Check sheet for the modelled part. Datum: model origin and axes. Units: mm. A direction names the side the tool comes from. Round coordinates to 2 decimals unless told otherwise and drop trailing zeros. Write each loop counter-clockwise with the first axis right and the second up, starting at its lowest first coordinate (ties: lowest second). Pieces come first, ordered by that corner, then holes. Notation, with made-up numbers: (9, -19) - (40, -19) arc R20 cw to (40, 17) - close; hole circle Ø1 at (42.25, 40.25). An arc over 180 degrees is marked (long way). Answer as a JSON object with one key per item and string values. Group by question number.
Item 1: Release check for a two-part mould opening along X. For faces 3 (the flat face through (4.28, -7.28, 15.86)), 4 (the flat face through (4.16, 7.35, 15.86)) record: pulls with the +X half, pulls with the -X half, needs draft (parallel to the pull), parting line crosses it, or undercut.
Item 2: Set-up check for faces 1 (the flat face through (-4.16, -7.35, 15.86)), 2 (the cylindrical face through (4.896, 2.03, 5.719)): record each of +Z, -Z, +X, -X, +Y, -Y from which the full face is reachable in a straight line by a thin tool's end or side.
Item 3: Gauge pin test, flat ends, axial feed: P1, Ø6.5, axis at x = 0, y = 0, coming from the +Z side; P2, Ø3, axis at x = -21, z = 17, coming from the -Y side (3 decimals); P3, Ø4, axis at y = -0.5, z = 14.5, coming from the +X side; P4, Ø6, axis at y = -20.5, z = 19.5, coming from the +X side. Record the tip position at first contact, or that the pin passes through.
Item 4: Thickness scan on line 1 (Y direction, x = 0, z = 16); line 2 (X direction, y = 0, z = 13); line 3 (Y direction, x = 0, z = 22). Record the ranges inside material, lowest first.
Item 5: Sectioned sample at B-B on z = 2.5. Record the boundary of the cut face in (x, y), plus the area to 3 significant figures.
Autodesk Inventor part; units mm, degrees
ref_plane "Work Plane1" through (-8.4437, 4.875, 0) normal (-0.5, -0.866, 0) x (0, 0, -1)
ref_plane "YZ Plane" through (0, 0, 0) normal (1, 0, 0) x (0, 1, 0)
ref_plane "XZ Plane" through (0, 0, 0) normal (0, 1, 0) x (-1, 0, 0)
sketch "Sketch1" plane through (0, 0, 0) normal (0, 0, 1) x (1, 0, 0)
  circle A0 centre (0, 0) radius 22.5
  circle A1 centre (0, 0) radius 32.5
  circle A2 centre (0, 0) radius 17.5
  circle A3 centre (0, 0) radius 12.8
  circle A4 centre (0, 0) radius 5.3
  circle A5 centre (0, 0) radius 9.75 construction
  line L0 (0, 9.75) -> (8.4437, 4.875)
  line L1 (8.4437, 4.875) -> (8.4437, -4.875)
  line L2 (8.4437, -4.875) -> (0, -9.75)
  line L3 (0, -9.75) -> (-8.4437, -4.875)
  line L4 (-8.4437, -4.875) -> (-8.4437, 4.875)
  line L5 (-8.4437, 4.875) -> (0, 9.75)
  line L6 (0, 9.75) -> (0, -9.75) construction
  dimension "bolt_head_hub_WAC" = 19.5
  dimension "wheel_diam" = 45
  dimension "d1" = 65
  dimension "d4" = 35
  dimension "d5" = 25.6
  dimension "hub_id" = 10.6
extrude "Extrusion1" add sketch "Sketch1" along normal blind 5 contours A0 | A1 | A2 | A3 | A4 | L0 L1 L2 L3 L4 L5
extrude "Extrusion2" add sketch "Sketch1" along normal blind 30 contours A0
extrude "Extrusion3" add sketch "Sketch1" along normal blind 20 contours A3 | L0 L1 L2 L3 L4 L5
extrude "Extrusion4" cut sketch "Sketch1" against normal blind 8.4 from surface at 20 contours L0 L1 L2 L3 L4 L5
extrude "Extrusion5" cut sketch "Sketch1" along normal up to surface (5 mm away) contours A4
fillet "Fillet1" radius 10 1 edges at (-22.5, 0, 5)
ref_plane "Work Plane1" through (-8.4437, 4.875, 0) normal (-0.5, -0.866, 0) x (0, 0, -1)
sketch "Sketch3" plane through (-8.4437, 4.875, 0) normal (-0.5, -0.866, 0) x (0, 0, -1)
  line L0 (-5, 22.55) -> (-20, 22.55)
  line L1 (-5, 27.25) -> (-5, -7.75)
  line L2 (-5, -3.05) -> (-5, 22.55)
  line L3 (-30, 27.25) -> (-5, 27.25)
  line L4 (-20, 22.55) -> (-5, 22.55)
  line L5 (-5, 22.55) -> (-5, 19.55)
  line L6 (-5, 19.55) -> (-20, 19.55)
  line L7 (-20, 19.55) -> (-20, 22.55)
  arc A0 (-20, 22.55) -> (-30, 27.25) centre (-30.9319, 12.279) ccw
  point P0 (0, 9.75)
  dimension "d18" = 3
  dimension "d21" = 15
extrude "Extrusion6" add sketch "Sketch3" along normal mid plane 3
pattern_circular "Circular Pattern1" count 4 over 360 about axis through (0, 0, -10) along (0, 0, 1) of "Extrusion6"
equation "\"bolt_head_hub_WAC\" = bolt_WAC + 2 * printer_tolerance"
equation "\"d1\" = wheel_diam + 2 * flange_extra"
equation "\"d4\" = wheel_diam - 2 * wheel_thick"
equation "\"d5\" = bolt_head_hub_WAC + 2 * bolt_head_hub_clearance"
equation "\"hub_id\" = bolt_od + 2 * printer_tolerance"
equation "\"d8\" = track_w + flange_w"
equation "\"d10\" = flange_w + hub_height"
equation "\"track_w\" = 25"
equation "\"wheel_thick\" = 5"
equation "\"bolt_head_hub_clearance\" = 3.05"
equation "\"hub_height\" = 15"
equation "\"bolt_head_thick\" = 6.4"
equation "\"bolt_WAC\" = 18.9"
equation "\"printer_tolerance\" = 0.3"
properties part number "test_wheel_v3"
Completed:
{
 "1": {"face 3": "undercut", "face 4": "undercut"},
 "2": {"face 1": "+Z", "face 2": "+Z, -Z"},
 "3": {"P1": "through", "P2": "y = -11.225", "P3": "x = 22.81", "P4": "x = 14.14"},
 "4": {"line 1": "-22.5 to -17.5, -12.8 to -9.75, 9.75 to 12.8, 17.5 to 22.5", "line 2": "-22.7 to -17.5, -12.8 to -8.44, 8.44 to 12.8, 17.5 to 22.7", "line 3": "-22.5 to -17.5, 17.5 to 22.5"},
 "5": {"outline": "circle Ø65 at (0, 0); hole circle Ø10.6 at (0, 0)", "area": "3,230 mm²"}
}
